Autodesk Inventor part; units mm, degrees
ref_plane "YZ Plane" through (0, 0, 0) normal (1, 0, 0) x (0, 1, 0)
ref_plane "XZ Plane" through (0, 0, 0) normal (0, 1, 0) x (-1, 0, 0)
ref_plane "XY Plane" through (0, 0, 0) normal (0, 0, 1) x (1, 0, 0)
sketch "Sketch2" plane through (0, 0, 0) normal (0, 0, 1) x (1, 0, 0)
  line L0 (-31.2032, 0) -> (39.8239, 0) construction
  line L1 (18.175, 9.4) -> (18.175, 11.1)
  line L2 (18.175, 11.1) -> (-18.175, 12)
  line L3 (-18.175, 12) -> (-18.175, 9.4)
  line L4 (0, 9.4) -> (0, 0) construction
  line L5 (6.825, 9.4) -> (6.825, 9.2)
  line L6 (6.825, 9.2) -> (7.325, 9.2)
  line L7 (7.325, 9.2) -> (7.325, 9.4)
  line L8 (-18.175, 9.4) -> (6.825, 9.4)
  line L9 (7.325, 9.4) -> (18.175, 9.4)
  line L10 (0, 11.55) -> (0, 9.4) construction
  dimension "d2" = 36.35
  dimension "d34" = 0.2
  dimension "d36" = 0.5
  dimension "d39" = 2.6
  dimension "d40" = 1.7
  dimension "d41" = 9.4
  dimension "d45" = 11.35
revolve "Revolution1" add sketch "Sketch2" angle 270 about axis through (-31.2032, 0, 0) along (1, 0, 0)
sketch "Sketch3" plane through (0, 0, 0) normal (0, 1, 0) x (-1, 0, 0)
  line L0 (18.175, 0) -> (18.175, -12)
  line L1 (18.175, -12) -> (18.175, -12)
  line L2 (18.175, -12) -> (18.175, 0)
  line L3 (18.175, 0) -> (18.175, 0)
  line L4 (-18.175, -9.4) -> (-18.175, -11.1)
  line L5 (-18.175, -11.1) -> (-18.175, 0)
  line L6 (-4.675, -5) -> (-4.675, 0)
  line L7 (7.175, -5) -> (-4.675, -5)
  line L8 (-18.175, -11.1) -> (18.175, -12)
  line L9 (18.175, -12) -> (-18.175, -11.1)
  line L10 (-4.675, 0) -> (-18.175, 0)
  line L11 (18.175, 0) -> (7.175, 0)
  line L12 (7.175, 0) -> (7.175, -5)
  dimension "d21" = 11
  dimension "d23" = 5
  dimension "d43" = 11.85
extrude "Extrusion1" cut sketch "Sketch3" against normal blind 200
sketch "Sketch4" plane through (0, 0, 0) normal (0, 1, 0) x (-1, 0, 0)
  line L0 (-18.175, 0) -> (18.175, 0)
  line L1 (7.175, 0) -> (-4.675, 0)
  line L2 (-4.675, 0) -> (-4.675, 6)
  line L3 (-4.675, 6) -> (7.175, 6)
  line L4 (7.175, 6) -> (7.175, 0)
  line L5 (18.175, 12) -> (18.175, 0)
  line L6 (-18.175, 11.1) -> (-18.175, 0)
  point P0 (-4.675, 0)
  dimension "d24" = 6
  dimension "d25" = 11
  dimension "d44" = 11.85
extrude "Extrusion2" cut sketch "Sketch4" along normal blind 200
chamfer "Chamfer1" distance 1.5 angle 45 1 edges at (18.175, 0, 11.1)
properties part number "PLASTIC_PART_big_one"
Check sheet for the modelled part. Datum: model origin and axes. Units: mm. A direction names the side the tool comes from. Give positions to 0.01 mm unless a question says otherwise; leave off trailing zeros. Order: outer loops, then holes, each group sorted by start corner. A loop starts at its lowest first (then second) coordinate and runs counter-clockwise, first axis right, second up. Notation, with made-up numbers: M 64,53 L 96,53 A19 ccw 96,64 Z; hole C -5.5,11.25 d6. An arc over 180 degrees is marked long. Answer in a Markdown table with one row per item. Add a question column.
Q1. Sectioned sample at D-D, the plane x = -15. Record the boundary of the cut face in (y, z), and give its area (3 significant figures).
Q2. Gauge pin test, flat ends, axial feed: pin 1 Ø3 at (x, y) = (-12.5, -10) entering from -Z; pin 2 Ø5 at (y, z) = (-8, 8.5) entering from +X (3 decimals); pin 3 Ø4 at (x, z) = (13.5, 4.5) entering from -Y; pin 4 Ø3 at (x, y) = (-0.5, 8) entering from -Z. Record the tip position at first contact, or that the pin passes through.
Q3. Sectioned sample at C-C, the plane x = -5. Record the boundary of the cut face in (y, z), and give its area (3 significant figures).
Q4. Thickness scan on L1, parallel to Y at x = -12, z = 6.25; L2, parallel to Y at x = -14, z = 6; L3, parallel to Y at x = -4, z = -0.5. Record the ranges inside material, lowest first.
Q5. Sectioned sample at A-A, the plane y = 0. Record the boundary of the cut face in (x, z) (3 decimals).
Q6. Sectioned sample at B-B, the plane z = 5. Count the separate pieces of the cut face and the enclosed holes in it, and give its area (3 significant figures).
Q7. Access from +Z, -Z, +X, -X, +Y, -Y to the whole of each face (thin tool, end or side, straight path). Record for faces 4 (the cylindrical face through (12.826, 0.207, 9.398)), 5 (the flat face through (-7.175, 10, 3)), 6 (the flat face through (4.675, -10, -3)), 7 (the flat face through (-13, -11, 0)).
Q8. Release check for a two-part mould opening along X. For faces 1 (the flat face through (4.675, 10, 3)), 2 (the cylindrical face through (7.078, 0.202, 9.198)), 3 (the flat face through (-7.175, -10, -2)) record: released by +X, released by -X, zero draft, split by the parting line, or undercut.
Verdict:
| question | item | result |
|---|---|---|
| 1 | outline | M -11.92,0 L -9.4,0 A9.4 cw 9.4,0 L 11.92,0 A11.92 ccw Z |
| 1 | area | 84.4 mm² |
| 2 | pin 1 | z = 0 |
| 2 | pin 2 | x = 18.175 |
| 2 | pin 3 | y = -10.94 |
| 2 | pin 4 | z = 6 |
| 3 | outline | M -10.55,-5 L -7.96,-5 A9.4 cw 7.24,6 L 10.01,6 A11.67 ccw Z |
| 3 | area | 72.6 mm² |
| 4 | L1 | -10.06 to -7.02, 7.02 to 10.06 |
| 4 | L2 | -10.27 to -7.24, 7.24 to 10.27 |
| 4 | L3 | -11.64 to -9.39 |
| 5 | outline | M -18.175,9.4 L 6.825,9.4 L 6.825,9.2 L 7.325,9.2 L 7.325,9.4 L 18.175,9.4 L 18.175,9.6 L 16.675,11.137 L -18.175,12 Z |
| 6 | separate pieces | 3 |
| 6 | enclosed holes | 0 |
| 6 | area | 146 mm² |
| 7 | face 4 | -Z, +X |
| 7 | face 5 | -Z, +Y |
| 7 | face 6 | -Z, +X, +Y, -Y |
| 7 | face 7 | -Z, -X, +Y, -Y |
| 8 | face 1 | undercut |
| 8 | face 2 | zero draft |
| 8 | face 3 | released by -X |
